from build123d import *

# Parameters (mm, degrees)
F2_DEPTH = 6.35
F1_W     = 1.778
F1_H     = 3.048
F1_H_2   = 5.842
F1_W_2   = 0.762
F5_DEPTH = 12.7
F6_DEPTH = 2.54


# Not quite as in the source:
# - a pattern or mirror of a feature is missing from the dataset's text; its kind, count and spacing are read off the source's solid
# - a feature names something its author has since deleted; it is built from what else it names


with BuildPart() as f2:
    # F0 (on Top) → F2 (new body)
    with BuildSketch(Plane.XY):
        with BuildLine():
            ThreePointArc((-14.5509208863, -2.5399817128), (-14.1547428746, -1.2973564714), (-14.0208, 0))
            ThreePointArc((-14.0208, 0), (-14.1547428746, 1.2973564714), (-14.5509208863, 2.5399817128))
            ThreePointArc((-14.5509208863, 2.5399817128), (-16.0448887373, 4.6485472727), (-18.2552900028, 5.9872462328))
            ThreePointArc((-18.2552900028, 5.9872462328), (-26.7208, 0), (-18.2552900028, -5.9872462328))
            ThreePointArc((-18.2552900028, -5.9872462328), (-16.0448887373, -4.6485472727), (-14.5509208863, -2.5399817128))
        make_face()
        with BuildLine():
            ThreePointArc((-18.2552900028, 5.9872462328), (-16.0448887373, 4.6485472727), (-14.5509208863, 2.5399817128))
            add(Edge.make_bspline(
                [(0, 1.524), (-9.0764431036, 1.3546369813), (-7.8380626316, 1.8652065321), (-14.5509208863, 2.5399817128)],
                knots=[0, 0, 0, 0, 14.5863469546, 14.5863469546, 14.5863469546, 14.5863469546], degree=3))
            add(Edge.make_bspline(
                [(0, 1.524), (9.0764431036, 1.3546369813), (7.8380626316, 1.8652065321), (14.5509208863, 2.5399817128)],
                knots=[0, 0, 0, 0, 14.5863469546, 14.5863469546, 14.5863469546, 14.5863469546], degree=3))
            ThreePointArc((14.5509208863, 2.5399817128), (16.0448887373, 4.6485472727), (18.2552900028, 5.9872462328))
            add(Edge.make_bspline(
                [(0, 2.54), (8.1250406802, 3.246476237), (11.4529688686, 3.5837408809), (18.2552900028, 5.9872462328)],
                knots=[0, 0, 0, 0, 18.5779202193, 18.5779202193, 18.5779202193, 18.5779202193], degree=3))
            add(Edge.make_bspline(
                [(0, 2.54), (-8.1250406802, 3.246476237), (-11.4529688686, 3.5837408809), (-18.2552900028, 5.9872462328)],
                knots=[0, 0, 0, 0, 18.5779202193, 18.5779202193, 18.5779202193, 18.5779202193], degree=3))
        make_face()
        with BuildLine():
            add(Edge.make_bspline(
                [(0, -1.524), (-9.0764431036, -1.3546369813), (-7.8380626316, -1.8652065321), (-14.5509208863, -2.5399817128)],
                knots=[0, 0, 0, 0, 14.5863469546, 14.5863469546, 14.5863469546, 14.5863469546], degree=3))
            ThreePointArc((-14.5509208863, -2.5399817128), (-16.0448887373, -4.6485472727), (-18.2552900028, -5.9872462328))
            add(Edge.make_bspline(
                [(0, -2.54), (-8.1250406802, -3.246476237), (-11.4529688686, -3.5837408809), (-18.2552900028, -5.9872462328)],
                knots=[0, 0, 0, 0, 18.5779202193, 18.5779202193, 18.5779202193, 18.5779202193], degree=3))
            add(Edge.make_bspline(
                [(0, -2.54), (8.1250406802, -3.246476237), (11.4529688686, -3.5837408809), (18.2552900028, -5.9872462328)],
                knots=[0, 0, 0, 0, 18.5779202193, 18.5779202193, 18.5779202193, 18.5779202193], degree=3))
            ThreePointArc((18.2552900028, -5.9872462328), (16.0448887373, -4.6485472727), (14.5509208863, -2.5399817128))
            add(Edge.make_bspline(
                [(0, -1.524), (9.0764431036, -1.3546369813), (7.8380626316, -1.8652065321), (14.5509208863, -2.5399817128)],
                knots=[0, 0, 0, 0, 14.5863469546, 14.5863469546, 14.5863469546, 14.5863469546], degree=3))
        make_face()
    extrude(amount=F2_DEPTH)

    # F2_copies: F2 across plane


with BuildPart() as f2_1:
    add(f2.part)
    add(f2.part.mirror(Plane(origin=(0, 0, 0), x_dir=(0, 0, 1), z_dir=(1, 0, 0))))

    # F1 (on Front) → F3 (revolve, cut)
    with BuildSketch(Plane.XZ):
        Polygon((20.344351037, 6.35), (20.344351037, 0), (24.459151037, 0), (23.824151037, 0.635), (23.824151037, 5.715), (24.459151037, 6.35), align=None)
    revolve(axis=Axis((20.344351037, 0, 3.175), (0, 0, 1)), mode=Mode.SUBTRACT)

    # F1 (on Front) → F4 (revolve)
    with BuildSketch(Plane.XZ):
        Polygon((-17.8308, 15.24), (-17.8308, 12.192), (-16.8148, 13.208), (-16.8148, 14.224), align=None)
        with Locations((-18.7198, 13.716)):
            Rectangle(F1_W, F1_H)
        with Locations((-22.0218, 13.716)):
            Rectangle(F1_W, F1_H)
        Polygon((-23.9268, 13.208), (-22.9108, 12.192), (-22.9108, 15.24), (-23.9268, 14.224), align=None)
        with Locations((-22.0218, 9.271)):
            Rectangle(F1_W, F1_H_2)
        with Locations((-18.7198, 9.271)):
            Rectangle(F1_W, F1_H_2)
    revolve(axis=Axis((-20.3708, 0, 10.795), (0, 0, 1)))

    # F1 (on Front) → F5 (cut, symmetric)
    with BuildSketch(Plane.XZ):
        with Locations((-19.9898, 13.716)):
            Rectangle(F1_W_2, F1_H)
        with Locations((-20.7518, 13.716)):
            Rectangle(F1_W_2, F1_H)
        with Locations((-19.9898, 9.271)):
            Rectangle(F1_W_2, F1_H_2)
        with Locations((-20.7518, 9.271)):
            Rectangle(F1_W_2, F1_H_2)
    extrude(amount=F5_DEPTH, both=True, mode=Mode.SUBTRACT)

    # F0 (on Top) → F6 (join)
    with BuildSketch(Plane.XY):
        with BuildLine():
            ThreePointArc((-14.5509208863, 2.5399817128), (-14.1547428746, 1.2973564714), (-14.0208, 0))
            ThreePointArc((-14.0208, 0), (-14.1547428746, -1.2973564714), (-14.5509208863, -2.5399817128))
            add(Edge.make_bspline(
                [(0, -1.524), (-9.0764431036, -1.3546369813), (-7.8380626316, -1.8652065321), (-14.5509208863, -2.5399817128)],
                knots=[0, 0, 0, 0, 14.5863469546, 14.5863469546, 14.5863469546, 14.5863469546], degree=3))
            add(Edge.make_bspline(
                [(0, -1.524), (9.0764431036, -1.3546369813), (7.8380626316, -1.8652065321), (14.5509208863, -2.5399817128)],
                knots=[0, 0, 0, 0, 14.5863469546, 14.5863469546, 14.5863469546, 14.5863469546], degree=3))
            ThreePointArc((14.5509208863, -2.5399817128), (14.0208, 0), (14.5509208863, 2.5399817128))
            add(Edge.make_bspline(
                [(0, 1.524), (9.0764431036, 1.3546369813), (7.8380626316, 1.8652065321), (14.5509208863, 2.5399817128)],
                knots=[0, 0, 0, 0, 14.5863469546, 14.5863469546, 14.5863469546, 14.5863469546], degree=3))
            add(Edge.make_bspline(
                [(0, 1.524), (-9.0764431036, 1.3546369813), (-7.8380626316, 1.8652065321), (-14.5509208863, 2.5399817128)],
                knots=[0, 0, 0, 0, 14.5863469546, 14.5863469546, 14.5863469546, 14.5863469546], degree=3))
        make_face()
    extrude(amount=F6_DEPTH)


solid = f2_1.part
Source: CAD feature listing. Evaluate the final solid. Frame: model axes, mm. A direction names the side the tool comes from. Round coordinates to 2 decimals unless told otherwise and drop trailing zeros. Write each loop counter-clockwise with the first axis right and the second up, starting at its lowest first coordinate (ties: lowest second). Pieces come first, ordered by that corner, then holes. Notation, with made-up numbers: M -36,82 L 1,82 A25 cw 1,117 Z; hole C 20,29 d11. An arc over 180 degrees is marked long. One line per item, written item: value. Start each with the question number.
Item 1: Pin query (flat end, axial travel): pin 1 (6.5 mm diameter, centred on x = -12.5, y = -2.5, fed in from +Z); pin 2 (7.5 mm diameter, centred on y = -1.5, z = 10, fed in from +X); pin 3 (3 mm diameter, centred on y = -3.5, z = 12.5, fed in from +X). Return the tip coordinate at first contact, or that it passes through.
Item 2: Set-up query: faces 1 (the cylindrical face through (-16.815, -0.067, 13.723)), 2 (the conical face through (-23.09, 0.05, 12.37)), 3 (the cylindrical face through (-23.926, 0.067, 13.723)), 4 (the flat face through (0, 0, 2.54)), 5 (the flat face through (-21.133, 0, 11)). Return all of +Z, -Z, +X, -X, +Y, -Y with unobstructed straight access to the full face (end or side cutting, diameter ignored); none if empty.
Item 3: Mould query, pull axis X, two halves, no side actions, for faces 6 (the flat face through (-19.609, 0, 11)), 7 (the conical face through (-17.655, -0.052, 12.368)), 8 (the flat face through (-6, 0, 0)), 9 (the cylindrical face through (-26.72, 0.17, 3.13)). Classes: pulls with the +X half, pulls with the -X half, needs draft (parallel to the pull), parting line crosses it, or undercut.
Item 4: Section query A-A (z = 10.25). Return the cut outline in (x, y).
Item 5: Ray query, L1, parallel to Z at x = -8.5, y = -2.25; L2, parallel to Y at x = 21, z = 5.5; L3, parallel to X at y = -0.5, z = 7.25. Return the intervals inside material, ascending. Write a range as from..to.
Result set:
1. pin 1: stops at z = 6.35
1. pin 2: stops at x = 26.69
1. pin 3: stops at x = -17.56
2. face 1: +Z, +X
2. face 2: -X
2. face 3: +Z, -X
2. face 4: +Z
2. face 5: +Z, +Y, -Y
3. face 6: undercut
3. face 7: pulls with the +X half
3. face 8: needs draft
3. face 9: undercut
4. outline: M -21.13,-2.42 L -21.13,2.42 A2.54 ccw Z; M -19.61,-2.42 A2.54 ccw -19.61,2.42 Z
5. L1: z = 0..6.35
5. L2: y = -6.32..-3.42, 3.42..6.32
5. L3: x = -22.86..-21.13, -19.61..-17.88
